```python
from build123d import *

# Parameters (mm, degrees)
BOSS_EXTRUDE1_DEPTH     = 50
FILLET1_R               = 2.54
FILLET2_R               = 5.715
SKETCH2_R               = 8.8
SKETCH2_R_2             = 2
CUT_EXTRUDE1_DEPTH      = 1
CUT_EXTRUDE1_DEPTH_BACK = 53
SKETCH4_R               = 3.175
CUT_EXTRUDE2_DEPTH      = 1
CUT_EXTRUDE2_DEPTH_BACK = 53


with BuildPart() as part:
    # Sketch1 → Boss-Extrude1 (new body)
    with BuildSketch(Plane(origin=(0, 0, 0), x_dir=(0, 0, -1), z_dir=(1, 0, 0))):
        Polygon((0, 0), (0, -52), (52, -52), (52, -48.825), (3.175, -48.825), (3.175, 0), align=None)
    extrude(amount=BOSS_EXTRUDE1_DEPTH)

    # Fillet1
    fillet1_edges = [part.edges().sort_by_distance(p)[0] for p in [
        (25, -48.825, -3.175),
    ]]
    fillet(fillet1_edges, radius=FILLET1_R)

    # Fillet2
    fillet2_edges = [part.edges().sort_by_distance(p)[0] for p in [
        (25, -52, 0),
    ]]
    fillet(fillet2_edges, radius=FILLET2_R)

    # Sketch2 → Cut-Extrude1 (cut, two sides)
    with BuildSketch(Plane.XY) as cut_extrude1_sk:
        with Locations((25, -24)):
            Circle(SKETCH2_R)
        with Locations((10.5, -24)):
            Circle(SKETCH2_R_2)
        with Locations((39.5, -24)):
            Circle(SKETCH2_R_2)
    extrude(amount=CUT_EXTRUDE1_DEPTH, mode=Mode.SUBTRACT)
    extrude(cut_extrude1_sk.sketch, amount=-CUT_EXTRUDE1_DEPTH_BACK, mode=Mode.SUBTRACT)

    # Sketch4 → Cut-Extrude2 (cut, two sides)
    with BuildSketch(Plane.XZ.offset(52)) as cut_extrude2_sk:
        with Locations((13.57, -27.94)):
            Circle(SKETCH4_R)
        with Locations((36.43, -27.94)):
            Circle(SKETCH4_R)
        with Locations((25, -12.7)):
            Circle(SKETCH4_R)
    extrude(amount=CUT_EXTRUDE2_DEPTH, mode=Mode.SUBTRACT)
    extrude(cut_extrude2_sk.sketch, amount=-CUT_EXTRUDE2_DEPTH_BACK, mode=Mode.SUBTRACT)


solid = part.part
```
Here's how the part is built. I have some questions about the finished solid (model axes, mm). A direction names the side the tool comes from. Give positions to 0.01 mm unless a question says otherwise; leave off trailing zeros. Write each loop counter-clockwise with the first axis right and the second up, starting at its lowest first coordinate (ties: lowest second). Pieces come first, ordered by that corner, then holes. Notation, with made-up numbers: M -18.75,12.5 L 29.25,12.5 A7 cw 29.25,17.5 Z; hole C 0,-4 d6. An arc over 180 degrees is marked long. Put each result on its own line as item: value. Start each with the question number.
Item 1: Will these pins go through, and if not, where does the flat tip stop? pin 1 (2 mm diameter, centred on x = 33, y = -20, fed in from -Z) (3 decimals); pin 2 (14 mm diameter, centred on x = 31, z = -36, fed in from +Y) (3 decimals); pin 3 (10.5 mm diameter, centred on x = 25, y = -24, fed in from +Z); pin 4 (10 mm diameter, centred on x = 40.5, z = -9.5, fed in from +Y).
Item 2: If we section it at C-C, the plane z = -12.7: Write out the boundary of the cut face in (x, y) (3 decimals).
Item 3: If we section it at A-A, the plane x = 25: Write out the boundary of the cut face in (y, z) (3 decimals).
Item 4: If we section it at B-B, the plane y = -24: Write out the boundary of the cut face in (x, z) (3 decimals), then the cut area to 3 significant figures.
Item 5: On a 3-axis mill with a long thin cutter (end or side, diameter ignored), from which of +Z, -Z, +X, -X, +Y, -Y can I reach the whole of each face in a straight line? I mean faces 4 (the cylindrical face through (25.35, -50.37, -1.72)), 5 (the flat face through (25, -34, -3.175)). Say none if no direction works.
Item 6: If we section it at D-D, the plane x = 13.57: Write out the boundary of the cut face in (y, z) (3 decimals), then the cut area to 3 significant figures.
Item 7: I need wall thicknesses on L1, parallel to X at y = -50, z = -27; L2, parallel to Y at x = 20.5, z = -39.5 (3 decimals); L3, parallel to Z at x = 41, y = -26 (3 decimals). Which ranges of each line are inside material? Lowest first, please. Write a range as from..to.
Item 8: Thinking about a two-plate mould opening in X: for faces 1 (the cylindrical face through (9.026, -22.648, -1.565)), 2 (the flat face through (25, -50, -52)), 3 (the flat face through (50, -37, -3)), which applies, +X half, -X half, draft (parallel to the pull), parting line (faces both ways), or undercut?
Values:
1. pin 1: z = -3.175
1. pin 2: y = -48.825
1. pin 3: through
1. pin 4: y = -48.52
2. outline: M 0,-52 L 21.825,-52 L 21.825,-48.825 L 0,-48.825 Z; M 28.175,-52 L 50,-52 L 50,-48.825 L 28.175,-48.825 Z
3. outline: M -52,-52 L -48.825,-52 L -48.825,-15.875 L -52,-15.875 Z; M -52,-9.525 L -48.825,-9.525 L -48.825,-5.715 A2.54 cw -46.285,-3.175 L -32.8,-3.175 L -32.8,0 L -46.285,0 A5.715 ccw -52,-5.715 Z; M -15.2,-3.175 L 0,-3.175 L 0,0 L -15.2,0 Z
4. outline: M 0,-3.175 L 8.5,-3.175 L 8.5,0 L 0,0 Z; M 12.5,-3.175 L 16.2,-3.175 L 16.2,0 L 12.5,0 Z; M 33.8,-3.175 L 37.5,-3.175 L 37.5,0 L 33.8,0 Z; M 41.5,-3.175 L 50,-3.175 L 50,0 L 41.5,0 Z
4. area: 77.5 mm²
5. face 4: +Z, +X, -X, -Y
5. face 5: -Z, +X, -X, +Y
6. outline: M -52,-52 L -48.825,-52 L -48.825,-31.115 L -52,-31.115 Z; M -52,-24.765 L -48.825,-24.765 L -48.825,-5.715 A2.54 cw -46.285,-3.175 L 0,-3.175 L 0,0 L -46.285,0 A5.715 ccw -52,-5.715 Z
6. area: 294 mm²
7. L1: 0..10.54, 16.6..33.4, 39.46..50
7. L2: -52..-48.825
7. L3: -3.175..0
8. face 1: undercut
8. face 2: draft
8. face 3: +X half
